Print and shaded views of the part. All mm, measured from the part's lowest x, y and z. Give positions to 0.01 mm unless a question says otherwise; leave off trailing zeros. Loops run counter-clockwise (first coordinate to the right, second up) from the corner with the lowest first, then second, coordinate; pieces in that order, holes last. Notation, with made-up numbers: (29, -2.5) - (51, -2.5) arc R29 cw to (51, 28.5) - close; hole circle Ø11 at (38.5, -19). An arc over 180 degrees is marked (long way). Return JSON: item names as keys, results as strings.
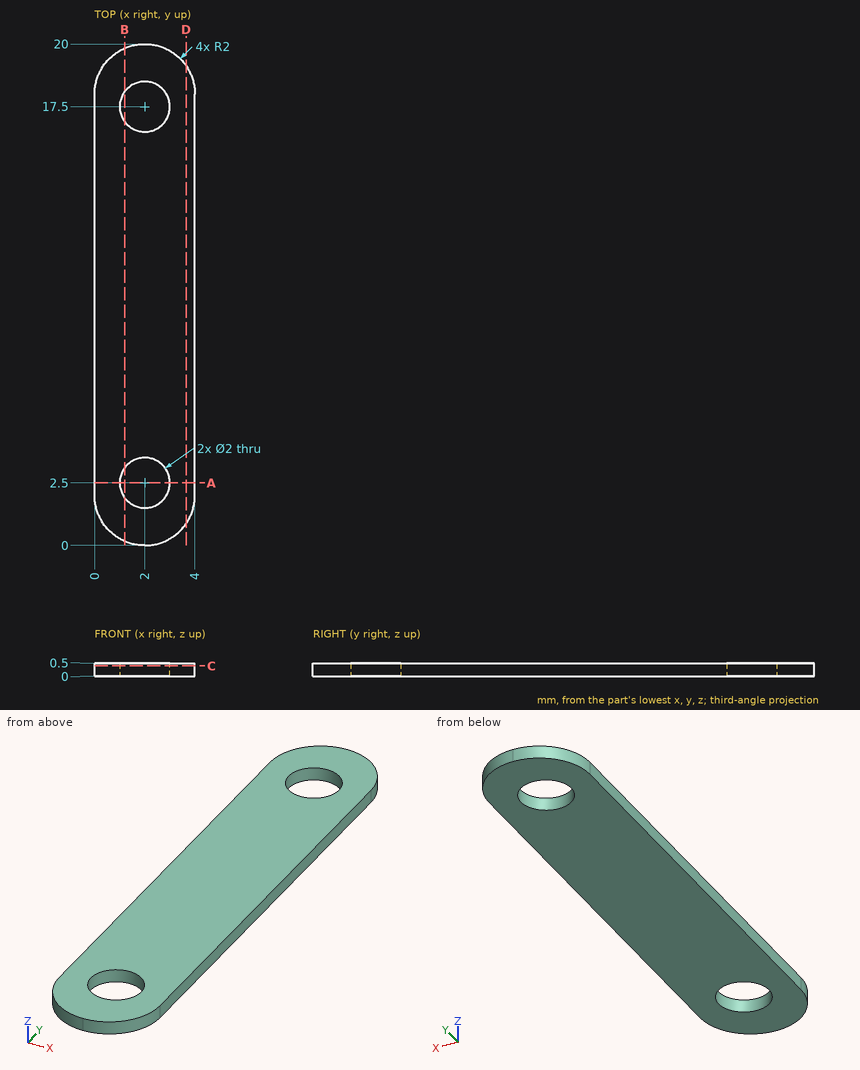
1. Cut at D-D, the plane x = 3.65. Write the cut outline in (y, z).
Values follow:
{"outline": "(0.87, 0) - (19.13, 0) - (19.13, 0.5) - (0.87, 0.5) - close"}
2. Cut at C-C, the plane z = 0.4. Give the number of separate pieces and of enclosed holes in the cut face, plus the area to 3 significant figures.
Values follow:
{"separate pieces": "1", "enclosed holes": "2", "area": "70.3 mm²"}
3. Cut at B-B, the plane x = 1.2. Write the cut outline in (y, z).
Values follow:
{"outline": "(0.17, 0) - (1.9, 0) - (1.9, 0.5) - (0.17, 0.5) - close; (3.1, 0) - (16.9, 0) - (16.9, 0.5) - (3.1, 0.5) - close; (18.1, 0) - (19.83, 0) - (19.83, 0.5) - (18.1, 0.5) - close"}
4. Cut at A-A, the plane y = 2.5. Write the cut outline in (x, z), plus the area to 3 significant figures.
Values follow:
{"outline": "(0, 0) - (1, 0) - (1, 0.5) - (0, 0.5) - close; (3, 0) - (4, 0) - (4, 0.5) - (3, 0.5) - close", "area": "1.00 mm²"}
5. Drill centre lines: probe 1 along Y at (x, z) = (2.75, 0.25); probe 2 along Y at (x, z) = (1.8, 0.1); probe 3 along X at (y, z) = (17, 0.2). Where is each one in solid material? Low to high.
Values follow:
{"probe 1": "y = 0.15 to 1.84, 3.16 to 16.84, 18.16 to 19.85", "probe 2": "y = 0.01 to 1.52, 3.48 to 16.52, 18.48 to 19.99", "probe 3": "x = 0 to 1.13, 2.87 to 4"}
